Input: part model. Units: mm. Frame: model coordinates. A direction names the side the tool comes from. Coordinates: 2 decimals unless noted, no trailing zeros. Write each loop counter-clockwise with the first axis right and the second up, starting at its lowest first coordinate (ties: lowest second). Pieces come first, ordered by that corner, then holes.
from build123d import *

# Parameters (mm, degrees)
EXTRUDE_2_DEPTH    = 6.2
HOLE_WIZARD_M3_1_D = 2.5


with BuildPart() as part:
    # 草图1 → 凸台-拉伸2 (new body)
    with BuildSketch(Plane.XY):
        Polygon((45, 5), (0, 5), (0, 0), (19.924787558, 0), (19.924787558, -2), (45, -2), align=None)
        with BuildLine():
            Line((29, -0.75), (41, -0.75))
            ThreePointArc((41, -0.75), (43.25, 1.5), (41, 3.75))
            Line((41, 3.75), (29, 3.75))
            ThreePointArc((29, 3.75), (26.75, 1.5), (29, -0.75))
        make_face(mode=Mode.SUBTRACT)
    extrude(amount=EXTRUDE_2_DEPTH)

    # M3 螺纹孔1 (through all)
    with Locations(Plane(origin=(0, -2, 0), x_dir=(-1, 0, 0), z_dir=(0, -1, 0))):
        with Locations((-22.5, -3.1), (-3.5, -3.1)):
            Hole(HOLE_WIZARD_M3_1_D / 2)


solid = part.part
Item 1: Section query C-C, the plane x = 3.5. Return loops of the section in (y, z).
Item 2: Section query D-D, the plane y = -1.5. Return loops of the section in (x, z).
Item 3: Material intervals for line 1 (Y direction, x = 34, z = 5.5); line 2 (X direction, y = 1.75, z = 3.75); line 3 (Z direction, x = 3.5, y = 3.45), sorted ascending.
Item 4: Section query A-A, the plane z = 3.1. Return loops of the section in (x, y).
Item 5: Section query B-B, the plane y = 1.5. Return loops of the section in (x, z), then the cut area to 3 significant figures.
Item 6: Pin query (flat end, axial travel): pin 1 Ø1.6 at (y, z) = (-1.5, 3) entering from -X; pin 2 Ø3 at (x, z) = (13, 4.5) entering from -Y; pin 3 Ø2 at (x, z) = (22.5, 3.1) entering from -Y. Return the tip coordinate at first contact, or that it passes through.
Item 7: Access query for faces 1 (the face through (23.655, 1.549, 3.579)), 2 (the face through (10, 0, 3)), 3 (the face through (35, 3.75, 3)). Directions: +Z, -Z, +X, -X, +Y, -Y. A direction counts if a zero-diameter tool reaches every point of the face in a straight line with its end or side. Return the directions, or none.
Item 8: Pull-direction query (X, two-part tool) for faces 4 (the face through (22.8, 5, 1.7)), 5 (the face through (35, -0.75, 3)), 6 (the face through (19.925, -1, 3)); classes: released by +X, released by -X, zero draft, split by the parting line, or undercut.
The answers:
1. outline: (0, 0) - (5, 0) - (5, 1.85) - (0, 1.85) - close; (0, 4.35) - (5, 4.35) - (5, 6.2) - (0, 6.2) - close
2. outline: (19.92, 0) - (45, 0) - (45, 6.2) - (19.92, 6.2) - close; hole circle Ø2.5 at (22.5, 3.1)
3. line 1: y = -2 to -0.75, 3.75 to 5
3. line 2: x = 0 to 2.43, 4.57 to 21.43, 23.57 to 26.76, 43.24 to 45
3. line 3: z = 0 to 1.85, 4.35 to 6.2
4. outline: (0, 0) - (2.25, 0) - (2.25, 5) - (0, 5) - close; (4.75, 0) - (19.92, 0) - (19.92, -2) - (21.25, -2) - (21.25, 5) - (4.75, 5) - close; (23.75, -2) - (45, -2) - (45, 5) - (23.75, 5) - close; hole (29, -0.75) - (41, -0.75) arc R2.25 ccw to (41, 3.75) - (29, 3.75) arc R2.25 ccw to start
5. outline: (0, 0) - (26.75, 0) - (26.75, 6.2) - (0, 6.2) - close; (43.25, 0) - (45, 0) - (45, 6.2) - (43.25, 6.2) - close; hole circle Ø2.5 at (3.5, 3.1); hole circle Ø2.5 at (22.5, 3.1)
5. area: 167 mm2
6. pin 1: stops at x = 19.92
6. pin 2: stops at y = 0
6. pin 3: passes through
7. face 1: +Y, -Y
7. face 2: +Z, -Z, -X, -Y
7. face 3: +Z, -Z
8. face 4: zero draft
8. face 5: undercut
8. face 6: released by -X
